Study the drawing (mm; zero at the part's minimum x, y, z) and answer. A direction names the side the tool comes from. Round coordinates to 2 decimals unless told otherwise and drop trailing zeros. Loops run counter-clockwise (first coordinate to the right, second up) from the corner with the lowest first, then second, coordinate; pieces in that order, holes last. Notation, with made-up numbers: M 67.25,44.25 L 112.25,44.25 A27 cw 112.25,64.25 Z; hole C 15,-35 d6. An arc over 180 degrees is marked long. Put each result on its own line as item: value. Start each with the question number.
(1) Section B-B, the plane z = 0.85 is taken. Determine the outline of the cut face in (x, y).
(2) Section C-C, the plane y = 23.5 is taken. Determine the outline of the cut face in (x, z), then the cut area to 3 significant figures.
(3) Straight lines are drawn through the part: line 1 (Z direction, x = 57, y = 28); line 2 (Y direction, x = 51, z = 4.5); line 3 (Y direction, x = 86.5, z = 3.6). For each, find the intervals that lie inside material, in ascending order.
(4) Section A-A, the plane x = 13 is taken. Determine the outline of the cut face in (y, z), then the cut area to 3 significant figures.
(5) Flat-ended cylindrical pins translate along their axes: P1, Ø1.3, axis at x = 34.5, z = 0.5, coming from the +Y side; P2, Ø14, axis at x = 46.5, y = 10, coming from the +Z side; P3, Ø0.8, axis at x = 65.5, z = 4, coming from the -Y side. Find the tip coordinate at first contact, or state that the pin passes through.
(6) Which of the six approach directions +Z, -Z, +X, -X, +Y, -Y give full straight-line access (tool end or side, diameter ignored) to the marked faces 1 and 2?
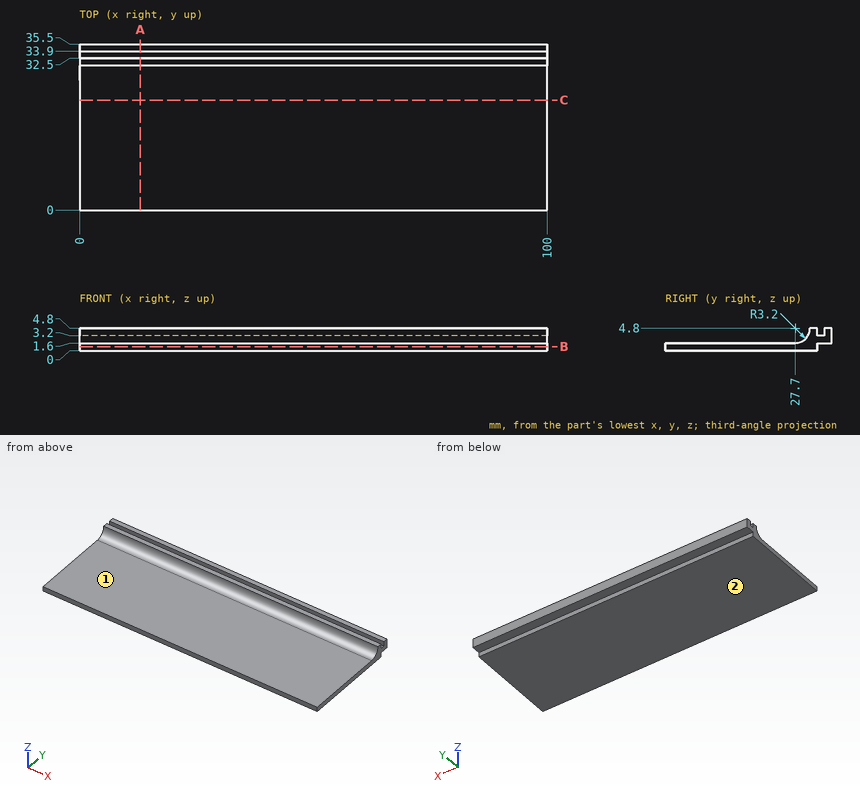
Recorded:
1. outline: M 0,0 L 100,0 L 100,32.5 L 0,32.5 Z
2. outline: M 0,0 L 100,0 L 100,1.6 L 0,1.6 Z
2. area: 160 mm²
3. line 1: z = 0 to 1.61
3. line 2: y = 30.89 to 32.5, 33.9 to 35.5
3. line 3: y = 30.67 to 32.5, 33.9 to 35.5
4. outline: M 0,0 L 32.5,0 L 32.5,1.6 L 35.5,1.6 L 35.5,4.8 L 33.9,4.8 L 33.9,3.2 L 32.5,3.2 L 32.5,4.8 L 30.9,4.8 A3.2 cw 27.7,1.6 L 0,1.6 Z
4. area: 66.7 mm²
5. P1: stops at y = 32.5
5. P2: stops at z = 1.6
5. P3: stops at y = 30.67
6. face 1: +Z, +X, -X, -Y
6. face 2: -Z, +X, -X, +Y, -Y
